For this review, take the finished solid that the model builds, in its own axes (mm). A direction names the side the tool comes from. Round coordinates to 2 decimals unless told otherwise and drop trailing zeros. Order: outer loops, then holes, each group sorted by start corner. A loop starts at its lowest first (then second) coordinate and runs counter-clockwise, first axis right, second up. Notation, with made-up numbers: M -21,49.5 L 34,49.5 A36 ccw 34,84.5 Z; hole C 46.5,-13 d6. An arc over 180 degrees is marked long. Use a Markdown table: item, result.
from build123d import *

# Parameters (mm, degrees)
SKETCH_3_R               = 45.9
EXTRUDE_3_DEPTH          = 2.6
SKETCH_4_R               = 45.9
SKETCH_4_R_2             = 35.9
EXTRUDE_4_DEPTH          = 6.8
SKETCH_5_R               = 2.85
CUT_EXTRUDE_3_DEPTH      = 6.8
SKETCH_13_R              = 10.4
SKETCH_13_R_2            = 2.85
EXTRUDE_5_DEPTH          = 11
SKETCH_14_R              = 10.4
SKETCH_14_R_2            = 2.85
EXTRUDE_6_DEPTH          = 3.8
SKETCH_17_R              = 9.9
CUT_EXTRUDE_5_DEPTH      = 67.321791291
PATTERN_CIRCULAR_1_COUNT = 5
SKETCH_19_R              = 1.8
CUT_EXTRUDE_6_DEPTH      = 67.321791291
PATTERN_CIRCULAR_2_COUNT = 5
SKETCH_20_R              = 47.9
SKETCH_20_R_2            = 45.9
EXTRUDE_7_DEPTH          = 6


with BuildPart() as part:
    # Sketch 3 → Extrude 3 (new, symmetric)
    with BuildSketch(Plane(origin=(0, 0, 0), x_dir=(0, 0, -1), z_dir=(1, 0, 0))):
        Circle(SKETCH_3_R)
    extrude(amount=EXTRUDE_3_DEPTH, both=True)

    # Sketch 4 → Extrude 4 (add, symmetric)
    with BuildSketch(Plane(origin=(0, 0, 0), x_dir=(0, 0, -1), z_dir=(1, 0, 0))):
        Circle(SKETCH_4_R)
        Circle(SKETCH_4_R_2, mode=Mode.SUBTRACT)
    extrude(amount=EXTRUDE_4_DEPTH, both=True)

    # Sketch 5 → Cut-Extrude 3 (cut, symmetric)
    with BuildSketch(Plane(origin=(0, 0, 0), x_dir=(0, 0, -1), z_dir=(1, 0, 0))):
        Circle(SKETCH_5_R)
    extrude(amount=CUT_EXTRUDE_3_DEPTH, both=True, mode=Mode.SUBTRACT)

    # Sketch 13 → Extrude 5 (add)
    with BuildSketch(Plane.ZY.offset(2.6)):
        with Locations(Location((0, 0, 0), (0, 0, 180))):
            Circle(SKETCH_13_R)
        with Locations(Location((0, 0, 0), (0, 0, 180))):
            Circle(SKETCH_13_R_2, mode=Mode.SUBTRACT)
    extrude(amount=EXTRUDE_5_DEPTH)

    # Sketch 14 → Extrude 6 (add)
    with BuildSketch(Plane(origin=(2.6, 0, 0), x_dir=(0, 0, -1), z_dir=(1, 0, 0))):
        Circle(SKETCH_14_R)
        Circle(SKETCH_14_R_2, mode=Mode.SUBTRACT)
    extrude(amount=EXTRUDE_6_DEPTH)

    # Sketch 17 → Cut-Extrude 5 (cut, symmetric)
    with BuildSketch(Plane(origin=(0, 0, 0), x_dir=(0, 0, -1), z_dir=(1, 0, 0))):
        with Locations((-13.45976737, 19.930809375)):
            Circle(SKETCH_17_R)
    cut_extrude_5 = extrude(amount=CUT_EXTRUDE_5_DEPTH, both=True, mode=Mode.SUBTRACT)

    # Pattern Circular 1: Cut-Extrude 5 ×5 about axis
    pattern_circular_1_axis = Axis((0, 0, 0), (1, 0, 0))
    for i in range(1, PATTERN_CIRCULAR_1_COUNT):
        add(cut_extrude_5.rotate(pattern_circular_1_axis, i * 360 / PATTERN_CIRCULAR_1_COUNT), mode=Mode.SUBTRACT)

    # Sketch 19 → Cut-Extrude 6 (cut, symmetric)
    with BuildSketch(Plane(origin=(0, 0, 0), x_dir=(0, 0, -1), z_dir=(1, 0, 0))):
        with Locations((-27.887163563, 11.720435504)):
            Circle(SKETCH_19_R)
    cut_extrude_6 = extrude(amount=CUT_EXTRUDE_6_DEPTH, both=True, mode=Mode.SUBTRACT)

    # Pattern Circular 2: Cut-Extrude 6 ×5 about axis
    pattern_circular_2_axis = Axis((0, 0, 0), (1, 0, 0))
    for i in range(1, PATTERN_CIRCULAR_2_COUNT):
        add(cut_extrude_6.rotate(pattern_circular_2_axis, i * 360 / PATTERN_CIRCULAR_2_COUNT), mode=Mode.SUBTRACT)

    # Sketch 20 → Extrude 7 (add, symmetric)
    with BuildSketch(Plane(origin=(0, 0, 0), x_dir=(0, 0, -1), z_dir=(1, 0, 0))):
        Circle(SKETCH_20_R)
        Circle(SKETCH_20_R_2, mode=Mode.SUBTRACT)
    extrude(amount=EXTRUDE_7_DEPTH, both=True)


solid = part.part
Q1. Add section C-C (y = -20). Write out the cut boundary in (x, z), then the cut area to 3 significant figures.
Determined:
| item | result |
|---|---|
| outline | M -6.8,-41.31 L -6,-41.31 L -6,-43.52 L 6,-43.52 L 6,-41.31 L 6.8,-41.31 L 6.8,-29.81 L 2.6,-29.81 L 2.6,-8.21 L -2.6,-8.21 L -2.6,-29.81 L -6.8,-29.81 Z; M -6.8,29.81 L -2.6,29.81 L -2.6,9.87 L 2.6,9.87 L 2.6,29.81 L 6.8,29.81 L 6.8,41.31 L 6,41.31 L 6,43.52 L -6,43.52 L -6,41.31 L -6.8,41.31 Z |
| area | 582 mm^2 |
Q2. Add section B-B (x = 0.5). Give the number of separate pieces and of enclosed holes in the cut face, then the cut area to 3 significant figures.
Determined:
| item | result |
|---|---|
| separate pieces | 1 |
| enclosed holes | 11 |
| area | 5,590 mm^2 |
Q3. Wall thickness on line 1 along Y through (x, z) = (-5.9, 0); line 2 along Y through (x, z) = (-8, 0); line 3 along Z through (x, y) = (4.5, -8.5): over which ranges is each line inside the solid? List them lowest first. Write a range as [from, to].
Determined:
| item | result |
|---|---|
| line 1 | y = [-47.9, -35.9], [-10.4, -2.85], [2.85, 10.4], [35.9, 47.9] |
| line 2 | y = [-10.4, -2.85], [2.85, 10.4] |
| line 3 | z = [-47.14, -34.88], [-5.99, 5.99], [34.88, 47.14] |
Q4. Add section A-A (y = 15). Write out the cut boundary in (x, z).
Determined:
| item | result |
|---|---|
| outline | M -6.8,-43.38 L -6,-43.38 L -6,-45.49 L 6,-45.49 L 6,-43.38 L 6.8,-43.38 L 6.8,-32.62 L 2.6,-32.62 L 2.6,-23.87 L -2.6,-23.87 L -2.6,-32.62 L -6.8,-32.62 Z; M -6.8,32.62 L -2.6,32.62 L -2.6,22.04 L 2.6,22.04 L 2.6,32.62 L 6.8,32.62 L 6.8,43.38 L 6,43.38 L 6,45.49 L -6,45.49 L -6,43.38 L -6.8,43.38 Z; M -2.6,-5.72 L 2.6,-5.72 L 2.6,4.88 L -2.6,4.88 Z |
Q5. Clearance check with flat-ended pins moving along their axes: pin 1 (2 mm diameter, centred on y = 0, z = 30.5, fed in from +X); pin 2 (3 mm diameter, centred on x = -3.5, y = -26.5, fed in from +Z); pin 3 (1 mm diameter, centred on y = 28, z = 2.5, fed in from -X). State where each tip first meets the part, or that it passes through.
Determined:
| item | result |
|---|---|
| pin 1 | stops at x = 2.6 |
| pin 2 | stops at z = 40.86 |
| pin 3 | stops at x = -2.6 |
Q6. Add section D-D (x = -10.5). Write out the cut boundary in (y, z).
Determined:
| item | result |
|---|---|
| outline | C 0,0 d20.8; hole C 0,0 d5.7 |
Q7. Machinability: for faces 1 (the flat face through (2.6, -7.5, -7.5)), 2 (the cylindrical face through (-3.74, -1.734, 2.262)), 3 (the cylindrical face through (-6.39, 13.79, -43.78)), which of the approach directions +Z, -Z, +X, -X, +Y, -Y give a long, thin tool a straight path to every point of the face, cutting with its end or side? Answer none if there is none.
Determined:
| item | result |
|---|---|
| face 1 | +X |
| face 2 | +X, -X |
| face 3 | -X |
